from build123d import *
from OCP.BRepFilletAPI import BRepFilletAPI_MakeFillet

# Parameters (mm, degrees)
SKETCH1_R                = 12
BOSS_EXTRUDE1_DEPTH      = 22
BOSS_EXTRUDE1_2_DEPTH    = 22
SKETCH1_3_W              = 60
SKETCH1_3_H              = 60
BOSS_EXTRUDE2_DEPTH      = 74
BOSS_EXTRUDE3_DEPTH      = 22
BOSS_EXTRUDE3_DEPTH_BACK = 44
SKETCH1_4_W              = 44
SKETCH1_4_H              = 20
FILLET1_R                = 30
FILLET1_R_2              = 22
CUT_EXTRUDE1_DEPTH       = 131.387882873
CUT_EXTRUDE1_DEPTH_BACK  = 131.387882873
SKETCH2_R                = 12
SKETCH2_R_2              = 8


with BuildPart() as part:
    # Sketch1 → Boss-Extrude1 (new body)
    with BuildSketch(Plane(origin=(0, 0, 0), x_dir=(1, 0, 0), z_dir=(0, 1, 0))):
        with BuildLine():
            Line((-65, -30), (-30, -30))
            Line((-30, -30), (-30, 30))
            Line((-30, 30), (-65, 30))
            ThreePointArc((-65, 30), (-95, 0), (-65, -30))
        make_face()
        with Locations(Location((-65, 0, 0), (0, 0, 270))):
            Circle(SKETCH1_R, mode=Mode.SUBTRACT)
    extrude(amount=BOSS_EXTRUDE1_DEPTH)



with BuildPart() as body_2:
    # Sketch1 → Boss-Extrude1 2 (new body)
    with BuildSketch(Plane(origin=(0, 0, 0), x_dir=(1, 0, 0), z_dir=(0, 1, 0))):
        with BuildLine():
            Line((51, -30), (95, -30))
            Line((95, -30), (95, 0))
            ThreePointArc((95, 0), (86.213203436, 21.213203436), (65, 30))
            Line((65, 30), (30, 30))
            Line((30, 30), (30, -30))
            Line((30, -30), (51, -30))
        make_face()
        with Locations(Location((65, 0, 0), (0, 0, 270))):
            Circle(SKETCH1_R, mode=Mode.SUBTRACT)
    extrude(amount=BOSS_EXTRUDE1_2_DEPTH)


with BuildPart() as part_1:
    add(part.part)

    add(body_2.part)  # Boss-Extrude2 merges body 2
    # Sketch1<3> → Boss-Extrude2 (add)
    with BuildSketch(Plane(origin=(0, 0, 0), x_dir=(1, 0, 0), z_dir=(0, 1, 0))):
        Rectangle(SKETCH1_3_W, SKETCH1_3_H)
    extrude(amount=BOSS_EXTRUDE2_DEPTH)

    # Sketch1<4> → Boss-Extrude3 (add, two sides: drawn at the far end of the back side and taken through both)
    with BuildSketch(Plane(origin=(0, 0, 0), x_dir=(1, 0, 0), z_dir=(0, 1, 0)).offset(-BOSS_EXTRUDE3_DEPTH_BACK)):
        with Locations((73, -40)):
            Rectangle(SKETCH1_4_W, SKETCH1_4_H)
    extrude(amount=BOSS_EXTRUDE3_DEPTH + BOSS_EXTRUDE3_DEPTH_BACK)

    # Fillet1
    fillet1_edges_1 = [part_1.edges().sort_by_distance(p)[0] for p in [
        (30, 74, 0),
        (-30, 74, 0),
    ]]
    fillet1_edges_2 = [part_1.edges().sort_by_distance(p)[0] for p in [
        (95, -44, 40),
        (51, -44, 40),
    ]]
    fillet1 = BRepFilletAPI_MakeFillet(part_1.part.solid().wrapped)
    for e in fillet1_edges_1:
        fillet1.Add(FILLET1_R - 0.0001, e.wrapped)
    for e in fillet1_edges_2:
        fillet1.Add(FILLET1_R_2 - 0.0001, e.wrapped)
    add(Compound.cast(fillet1.Shape()), mode=Mode.REPLACE)  # a hair under: the kernel refuses the full size

    # Sketch2 → Cut-Extrude1 (cut, two sides: drawn at the far end of the back side and taken through both)
    with BuildSketch(Plane.XY.offset(-CUT_EXTRUDE1_DEPTH_BACK)):
        with Locations((0, 44)):
            Circle(SKETCH2_R)
        with Locations((73, -22)):
            Circle(SKETCH2_R_2)
    extrude(amount=CUT_EXTRUDE1_DEPTH + CUT_EXTRUDE1_DEPTH_BACK, mode=Mode.SUBTRACT)


solid = part_1.part
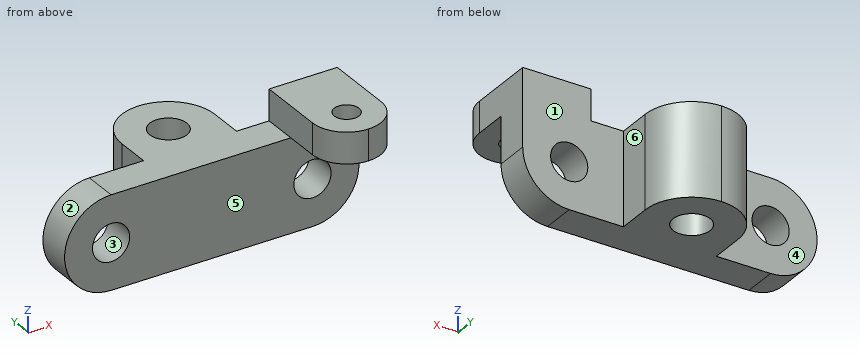
Design review of the part built by this model. Coordinates are the model's own, in mm. Face numbers are marked on the shaded views. A direction names the side the tool comes from. Coordinates: 2 decimals unless noted, no trailing zeros. Write each loop counter-clockwise with the first axis right and the second up, starting at its lowest first coordinate (ties: lowest second). Pieces come first, ordered by that corner, then holes. Notation, with made-up numbers: (53, -34.75) - (77, -34.75) arc R16 cw to (77, -22.75) - close; hole circle Ø3 at (27, 78.5). An arc over 180 degrees is marked (long way). Use one line per item in the form item = value.
Q1. Consider section B-B (y = 40.5). Write out the cut boundary in (x, z), plus the area to 3 significant figures.
Taken from the geometry:
outline = (-30, -30) - (-11.48, -30) - (-11.48, 30) - (-30, 30) - close; (11.48, -30) - (30, -30) - (30, 30) - (11.48, 30) - close
area = 2,220 mm^2
Q2. Consider section A-A (z = -9). Count the separate pieces of the cut face and the enclosed holes in it, plus the area to 3 significant figures.
Taken from the geometry:
separate_pieces = 3
enclosed_holes = 1
area = 5,700 mm^2
Q3. Machinability: for the marked faces 4, 5 and 6, which of the approach directions +Z, -Z, +X, -X, +Y, -Y give a long, thin tool a straight path to every point of the face, cutting with its end or side? Answer none if there is none.
Taken from the geometry:
face_4 = +Z, -Z, -X, +Y
face_5 = -Z, +X, -X, -Y
face_6 = +Z, -Z, +X, +Y
Q4. Consider section D-D (x = 75). Write out the cut boundary in (y, z).
Taken from the geometry:
outline = (-43.91, 30) - (-29.75, 30) - (-29.75, 50) - (-43.91, 50) - close; (-14.25, 30) - (0, 30) - (0, 6.63) - (22, 6.63) - (22, 50) - (-14.25, 50) - close; (0, -28.28) - (22, -28.28) - (22, -6.63) - (0, -6.63) - close
Q5. The part is to be moulded in two halves that separate along Z. For the marked faces 1, 2 and 3, say which applies: +Z half, -Z half, draft (parallel to the pull), parting line (faces both ways), or undercut.
Taken from the geometry:
face_1 = draft
face_2 = parting line
face_3 = undercut
Q6. For probe 1 along X at (y, z) = (7, 0); probe 2 along X at (y, z) = (-22, 43); probe 3 along Y at (x, z) = (0, 2), list the stretches that pass through material, from the lowest coordinate up.
Taken from the geometry:
probe_1 = -95 to -77, -53 to 53, 77 to 95
probe_2 = 51 to 65, 81 to 95
probe_3 = 0 to 32, 56 to 74
Q7. Insertion check: pin 1 Ø3 at (x, z) = (8, -8) entering from +Y; pin 2 Ø4 at (x, z) = (17.5, 26.5) entering from -Y; pin 3 Ø22 at (x, y) = (17, 46) entering from +Z; pin 4 Ø10 at (y, z) = (-1.5, 15) entering from +X. Each pin has a flat end and moves straight along its axis. Give the tip position at first contact, or say it passes through.
Taken from the geometry:
pin_1 = 73.29
pin_2 = 0
pin_3 = 30
pin_4 = 95
